Verification items for the finished model (mm, model axes). A direction names the side the tool comes from. Round coordinates to 2 decimals unless told otherwise and drop trailing zeros. Write each loop counter-clockwise with the first axis right and the second up, starting at its lowest first coordinate (ties: lowest second). Pieces come first, ordered by that corner, then holes. Notation, with made-up numbers: (-23, 38.25) -> (8, 38.25) arc R32 cw to (8, 71.25) -> close; hole circle Ø6 at (59, 41.25). An arc over 180 degrees is marked (long way). Use CSV: the item, a comma, the result in double quotes.
```python
from build123d import *

# Parameters (mm, degrees)
F0_W           = 304.8
F0_H           = 203.2
F1_DEPTH       = 19.05
F2_W           = 228.6
F2_H           = 25.4
F3_DEPTH       = 19.051
F5_D           = 6.35
F7_D           = 12.7
F9_D           = 9.525
F9_CBORE_D     = 12.7
F9_CBORE_DEPTH = 12.7


with BuildPart() as f1:
    # F0 (on Front) → F1 (new body)
    with BuildSketch(Plane.XZ):
        with Locations((152.4, 101.6)):
            Rectangle(F0_W, F0_H)
    extrude(amount=F1_DEPTH)

    # F2 (on face) → F3 (cut, through all)
    with BuildSketch(Plane.XZ.offset(19.05)):
        with Locations((152.4, 12.7)):
            Rectangle(F2_W, F2_H)
    extrude(amount=-F3_DEPTH, mode=Mode.SUBTRACT)

    # F5 (through all)
    with Locations(Plane.XZ.offset(19.05)):
        with Locations((120.65, 38.1), (184.15, 38.1)):
            Hole(F5_D / 2)

    # F7 (through all)
    with Locations(Plane.XZ.offset(19.05)):
        with Locations((152.4, 105.6132)):
            Hole(F7_D / 2)

    # F9 (through all)
    with Locations(Plane.XZ.offset(19.05)):
        with Locations((19.05, 19.05), (19.05, 95.25), (285.75, 19.05), (285.75, 95.25)):
            CounterBoreHole(F9_D / 2, F9_CBORE_D / 2, F9_CBORE_DEPTH)


solid = f1.part
```
Q1. Section check D-D (z = 19.05). Record the cut outline in (x, y), plus the area to 3 significant figures.
Filled in:
outline,"(0, -19.05) -> (12.7, -19.05) -> (12.7, -6.35) -> (14.29, -6.35) -> (14.29, 0) -> (0, 0) -> close; (23.81, -6.35) -> (25.4, -6.35) -> (25.4, -19.05) -> (38.1, -19.05) -> (38.1, 0) -> (23.81, 0) -> close; (266.7, -19.05) -> (279.4, -19.05) -> (279.4, -6.35) -> (280.99, -6.35) -> (280.99, 0) -> (266.7, 0) -> close; (290.51, -6.35) -> (292.1, -6.35) -> (292.1, -19.05) -> (304.8, -19.05) -> (304.8, 0) -> (290.51, 0) -> close"
area,"1,010 mm²"
Q2. Section check C-C (x = 152.4). Record the cut outline in (y, z), plus the area to 3 significant figures.
Filled in:
outline,"(-19.05, 25.4) -> (0, 25.4) -> (0, 99.26) -> (-19.05, 99.26) -> close; (-19.05, 111.96) -> (0, 111.96) -> (0, 203.2) -> (-19.05, 203.2) -> close"
area,"3,150 mm²"
Q3. Access from +Z, -Z, +X, -X, +Y, -Y to the whole of each face (thin tool, end or side, straight path). Record for faces 5 (the flat face through (288, -6.35, 100)), 6 (the flat face through (151, -10, 25.4)), 7 (the flat face through (0, -9, 100)).
Filled in:
face 5,"-Y"
face 6,"-Z, +Y, -Y"
face 7,"+Z, -Z, -X, +Y, -Y"
Q4. Go/stop test with flat-tipped pins: P1, Ø1.5, axis at x = 70, y = -3.5, coming from the -Z side; P2, Ø10, axis at x = 285.75, z = 19.05, coming from the -Y side. Record where each tip stops, or that it passes through.
Filled in:
P1,"z = 25.4"
P2,"y = -6.35"
Q5. Material ranges on L1, parallel to Z at x = 285.75, y = -12.75; L2, parallel to X at y = -15.5, z = 95; L3, parallel to X at y = -9.75, z = 11, recorded low to high.
Filled in:
L1,"0 to 12.7, 25.4 to 88.9, 101.6 to 203.2"
L2,"0 to 12.7, 25.4 to 279.4, 292.1 to 304.8"
L3,"0 to 38.1, 266.7 to 304.8"
Q6. Section check B-B (z = 95.25). Record the cut outline in (x, y).
Filled in:
outline,"(0, -19.05) -> (12.7, -19.05) -> (12.7, -6.35) -> (14.29, -6.35) -> (14.29, 0) -> (0, 0) -> close; (23.81, -6.35) -> (25.4, -6.35) -> (25.4, -19.05) -> (279.4, -19.05) -> (279.4, -6.35) -> (280.99, -6.35) -> (280.99, 0) -> (23.81, 0) -> close; (290.51, -6.35) -> (292.1, -6.35) -> (292.1, -19.05) -> (304.8, -19.05) -> (304.8, 0) -> (290.51, 0) -> close"
Q7. Mould release check, pull along X, two halves, no side actions. Record for faces 1 (the flat face through (285, -9, 0)), 2 (the flat face through (304.8, -9, 100)), 3 (the cylindrical face through (19.67, -3.13, 99.97)), 4 (the cylindrical face through (17.67, -12.79, 89.05)): released by +X, released by -X, zero draft, split by the parting line, or undercut.
Filled in:
face 1,"zero draft"
face 2,"released by +X"
face 3,"undercut"
face 4,"undercut"
Q8. Section check A-A (x = 19.05). Record the cut outline in (y, z).
Filled in:
outline,"(-19.05, 0) -> (0, 0) -> (0, 14.29) -> (-6.35, 14.29) -> (-6.35, 12.7) -> (-19.05, 12.7) -> close; (-19.05, 25.4) -> (-6.35, 25.4) -> (-6.35, 23.81) -> (0, 23.81) -> (0, 90.49) -> (-6.35, 90.49) -> (-6.35, 88.9) -> (-19.05, 88.9) -> close; (-19.05, 101.6) -> (-6.35, 101.6) -> (-6.35, 100.01) -> (0, 100.01) -> (0, 203.2) -> (-19.05, 203.2) -> close"
